```python
from build123d import *

# Parameters (mm, degrees)
F0_R     = 10.95
F0_R_2   = 6.45
F1_DEPTH = 7
F2_R     = 5
F3_SIZE  = 2.5
F4_R     = 6.45
F4_R_2   = 5.85
F5_DEPTH = 1
F6_SIZE  = 0.7
F8_DEPTH = 25


with BuildPart() as f1:
    # F0 (on Top) → F1 (new body)
    with BuildSketch(Plane.XY):
        with BuildLine():
            Line((8.6602540378, 5), (14.6370370137, 18.538022945))
            ThreePointArc((14.6370370137, 18.538022945), (0, 41), (-14.6370370137, 18.538022945))
            Line((-14.6370370137, 18.538022945), (-8.6602540378, 5))
            Line((-8.6602540378, 5), (-23.3729173132, 3.4070344175))
            ThreePointArc((-23.3729173132, 3.4070344175), (-35.5070415552, -20.5), (-8.7358802995, -21.9450573625))
            Line((-8.7358802995, -21.9450573625), (0, -10))
            Line((0, -10), (8.7358802995, -21.9450573625))
            ThreePointArc((8.7358802995, -21.9450573625), (35.5070415552, -20.5), (23.3729173132, 3.4070344175))
            Line((23.3729173132, 3.4070344175), (8.6602540378, 5))
        make_face()
        with Locations((-21.6506350946, -12.5)):
            Circle(F0_R, mode=Mode.SUBTRACT)
        with Locations((21.6506350946, -12.5)):
            Circle(F0_R, mode=Mode.SUBTRACT)
        Circle(F0_R_2, mode=Mode.SUBTRACT)
        with Locations((0, 25)):
            Circle(F0_R, mode=Mode.SUBTRACT)
    extrude(amount=F1_DEPTH)

    # F2
    f2_edges = [f1.edges().sort_by_distance(p)[0] for p in [
        (0, -10, 3.5),
        (8.660254, 5, 3.5),
        (-8.660254, 5, 3.5),
    ]]
    fillet(f2_edges, radius=F2_R)

    # F3
    f3_edges = [f1.edges().sort_by_distance(p)[0] for p in [
        (-19.415113, 3.835553, 7),
        (-6.385871, -18.731758, 0),
        (19.415113, 3.835553, 0),
        (19.415113, 3.835553, 7),
        (11.665396, 6.735019, 0),
        (35.507042, -20.5, 0),
        (13.029243, 14.896205, 0),
        (6.385871, -18.731758, 0),
        (0, 41, 0),
        (0, -13.470039, 0),
        (-13.029243, 14.896205, 0),
        (-11.665396, 6.735019, 0),
        (-35.507042, -20.5, 0),
        (-19.415113, 3.835553, 0),
        (11.665396, 6.735019, 7),
        (35.507042, -20.5, 7),
        (13.029243, 14.896205, 7),
        (6.385871, -18.731758, 7),
        (0, 41, 7),
        (0, -13.470039, 7),
        (-13.029243, 14.896205, 7),
        (-6.385871, -18.731758, 7),
        (-11.665396, 6.735019, 7),
        (-35.507042, -20.5, 7),
    ]]
    chamfer(f3_edges, length=F3_SIZE)

    # F4 (on face) → F5 (join)
    with BuildSketch(Plane(origin=(0, 0, 0), x_dir=(1, 0, 0), z_dir=(0, 0, -1))):
        Circle(F4_R)
        Circle(F4_R_2, mode=Mode.SUBTRACT)
    extrude(amount=-F5_DEPTH)

    # F6
    f6_edges = [f1.edges().sort_by_distance(p)[0] for p in [
        (-6.45, 0, 7),
        (-32.600635, -12.5, 7),
        (10.700635, -12.5, 7),
        (-10.95, 25, 7),
        (-32.600635, -12.5, 0),
        (10.700635, -12.5, 0),
        (-10.95, 25, 0),
    ]]
    chamfer(f6_edges, length=F6_SIZE)

    # F7 (on face) → F8 (cut)
    with BuildSketch(Plane.XY.offset(7)):
        with BuildLine():
            ThreePointArc((-4.1486247409, -8.4906662141), (-8.1839400658, -4.725), (-9.4274450069, 0.6525186907))
            ThreePointArc((-9.4274450069, 0.6525186907), (-11.4491842198, -0.4430009845), (-13.6635486442, -1.0628259595))
            ThreePointArc((-13.6635486442, -1.0628259595), (-9.5695807118, -5.525), (-7.7522086028, -11.3015672519))
            ThreePointArc((-7.7522086028, -11.3015672519), (-6.1082422164, -9.6937838947), (-4.1486247409, -8.4906662141))
        make_face()
        with BuildLine():
            ThreePointArc((-5.278820266, 7.8381475234), (0, 9.45), (5.278820266, 7.8381475234))
            ThreePointArc((5.278820266, 7.8381475234), (5.3409420034, 10.1367848792), (5.9113400414, 12.3643932114))
            ThreePointArc((5.9113400414, 12.3643932114), (0, 11.05), (-5.9113400414, 12.3643932114))
            ThreePointArc((-5.9113400414, 12.3643932114), (-5.3409420034, 10.1367848792), (-5.278820266, 7.8381475234))
        make_face()
        with BuildLine():
            ThreePointArc((9.4274450069, 0.6525186907), (8.1839400658, -4.725), (4.1486247409, -8.4906662141))
            ThreePointArc((4.1486247409, -8.4906662141), (6.1082422164, -9.6937838947), (7.7522086028, -11.3015672519))
            ThreePointArc((7.7522086028, -11.3015672519), (9.5695807118, -5.525), (13.6635486442, -1.0628259595))
            ThreePointArc((13.6635486442, -1.0628259595), (11.4491842198, -0.4430009845), (9.4274450069, 0.6525186907))
        make_face()
    extrude(amount=-F8_DEPTH, mode=Mode.SUBTRACT)


solid = f1.part
```
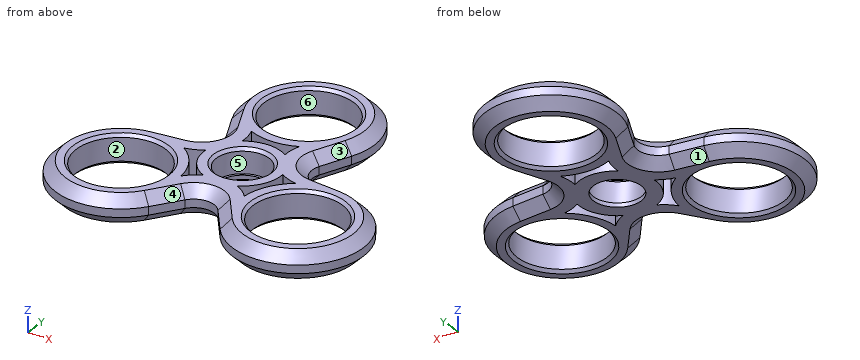
Part model, mm, in its own coordinate system. Face numbers are marked on the shaded views. A direction names the side the tool comes from. Coordinates: 2 decimals unless noted, no trailing zeros. Order: outer loops, then holes, each group sorted by start corner. A loop starts at its lowest first (then second) coordinate and runs counter-clockwise, first axis right, second up. Notation, with made-up numbers: (75, 15.5) - (130, 15.5) arc R19 ccw to (130, 22.5) - close; hole circle Ø4 at (27, 12). An arc over 180 degrees is marked (long way). Return JSON: item names as keys, results as strings. Group by question number.
Item 1: Cut at C-C (z = 3.5). List the corners of the cut face in (x, y), plus the area to 3 significant figures.
Item 2: Cut at A-A (y = 25). List the corners of the cut face in (x, z), plus the area to 3 significant figures.
Item 3: Pull direction X, two halves, no side cores. Call the marked faces 1, 2 and 3: pulls with the +X half, pulls with the -X half, needs draft (parallel to the pull), parting line crosses it, or undercut.
Item 4: Pin check, flat tips, straight feed: pin 1 (1.5 mm diameter, centred on y = -3, z = 2.5, fed in from -X); pin 2 (10.5 mm diameter, centred on x = 0, y = 0, fed in from -Z); pin 3 (1.5 mm diameter, centred on y = 11.5, z = 6, fed in from -X); pin 4 (1 mm diameter, centred on x = 24.5, z = 4, fed in from +Y). Stop position of each tip, or through.
Item 5: Cut at B-B (x = 0). State how many separate pieces and enclosed holes the cut face has, plus the area to 3 significant figures.
Item 6: Which spindle directions (+Z, -Z, +X, -X, +Y, -Y) get a long thin tool onto all of the face, cutting with end or side? Do the marked faces 4, 5 and 6. Say none if no direction does.
Item 7: Drill centre lines: probe 1 along Y at (x, z) = (0, 3.25); probe 2 along Y at (x, z) = (13, 4.75); probe 3 along Y at (x, z) = (-7.5, 3). Where is each one in solid material? Low to high. Write a range as from..to.
Check values:
{
 "1": {"outline": "(-23.37, 3.41) arc R16 ccw (long way) to (-8.74, -21.95) - (-4.04, -15.52) arc R5 cw to (4.04, -15.52) - (8.74, -21.95) arc R16 ccw (long way) to (23.37, 3.41) - (15.46, 4.26) arc R5 cw to (11.42, 11.25) - (14.64, 18.54) arc R16 ccw (long way) to (-14.64, 18.54) - (-11.42, 11.25) arc R5 cw to (-15.46, 4.26) - close; hole circle Ø21.9 at (-21.65, -12.5); hole (-13.66, -1.06) arc R13.95 cw to (-7.75, -11.3) arc R10.3 cw to (-4.15, -8.49) arc R9.45 cw to (-9.43, 0.65) arc R10.3 cw to start; hole circle Ø21.9 at (0, 25); hole circle Ø12.9 at (0, 0); hole (-5.91, 12.36) arc R10.3 cw to (-5.28, 7.84) arc R9.45 cw to (5.28, 7.84) arc R10.3 cw to (5.91, 12.36) arc R13.95 cw to start; hole (4.15, -8.49) arc R10.3 cw to (7.75, -11.3) arc R13.95 cw to (13.66, -1.06) arc R10.3 cw to (9.43, 0.65) arc R9.45 cw to start; hole circle Ø21.9 at (21.65, -12.5)", "area": "1,580 mm2"},
 "2": {"outline": "(-16, 2.5) - (-13.5, 0) - (-11.65, 0) - (-10.95, 0.7) - (-10.95, 6.3) - (-11.65, 7) - (-13.5, 7) - (-16, 4.5) - close; (10.95, 0.7) - (11.65, 0) - (13.5, 0) - (16, 2.5) - (16, 4.5) - (13.5, 7) - (11.65, 7) - (10.95, 6.3) - close", "area": "57.2 mm2"},
 "3": {"face 1": "pulls with the -X half", "face 2": "undercut", "face 3": "pulls with the +X half"},
 "4": {"pin 1": "stops at x = -35.05", "pin 2": "passes through", "pin 3": "stops at x = -10.77", "pin 4": "stops at y = 3.33"},
 "5": {"separate pieces": "4", "enclosed holes": "0", "area": "114 mm2"},
 "6": {"face 4": "+Z, -Y", "face 5": "+Z", "face 6": "+Z, -Z"},
 "7": {"probe 1": "y = -13.47..-6.45, 6.45..9.45, 11.05..14.05, 35.95..41", "probe 2": "y = -25.66..-19.21, -5.79..-1.56, -0.93..4.92, 15.45..33.89", "probe 3": "y = -20.26..-11, -5.75..17.02, 32.98..39.13"}
}
